from build123d import *

# Parameters (mm, degrees)
SKETCH1_R           = 1
SKETCH1_R_2         = 4.5
BOSS_EXTRUDE1_DEPTH = 2
SKETCH1_4_R         = 4.5
CUT_EXTRUDE1_DEPTH  = 1


with BuildPart() as part:
    # Sketch1 → Boss-Extrude1 (new body)
    with BuildSketch(Plane(origin=(0, 0, 0), x_dir=(1, 0, 0), z_dir=(0, 1, 0))):
        with BuildLine():
            Line((-6, 11), (6, 11))
            ThreePointArc((6, 11), (9.535533906, 9.535533906), (11, 6))
            Line((11, 6), (11, -6))
            ThreePointArc((11, -6), (9.535533906, -9.535533906), (6, -11))
            Line((6, -11), (-6, -11))
            ThreePointArc((-6, -11), (-9.535533906, -9.535533906), (-11, -6))
            Line((-11, -6), (-11, 6))
            ThreePointArc((-11, 6), (-9.535533906, 9.535533906), (-6, 11))
        make_face()
        with Locations((-6.992221877, 6.992221877)):
            Circle(SKETCH1_R, mode=Mode.SUBTRACT)
        with Locations((6.992221877, 6.992221877)):
            Circle(SKETCH1_R, mode=Mode.SUBTRACT)
        with Locations((6.992221877, -6.992221877)):
            Circle(SKETCH1_R, mode=Mode.SUBTRACT)
        with Locations((-6.992221877, -6.992221877)):
            Circle(SKETCH1_R, mode=Mode.SUBTRACT)
        Circle(SKETCH1_R_2, mode=Mode.SUBTRACT)
        with Locations((-6.363961031, 0)):
            Circle(SKETCH1_R, mode=Mode.SUBTRACT)
        with Locations((6.363961031, 0)):
            Circle(SKETCH1_R, mode=Mode.SUBTRACT)
    extrude(amount=BOSS_EXTRUDE1_DEPTH)

    # Sketch1_4 → Cut-Extrude1 (cut)
    with BuildSketch(Plane(origin=(0, 0, 0), x_dir=(1, 0, 0), z_dir=(0, 1, 0))):
        with BuildLine():
            Line((2.121320344, 9.192388155), (9.192388155, 2.121320344))
            ThreePointArc((9.192388155, 2.121320344), (10.071067812, 0), (9.192388155, -2.121320344))
            Line((9.192388155, -2.121320344), (2.121320344, -9.192388155))
            ThreePointArc((2.121320344, -9.192388155), (0, -10.071067812), (-2.121320344, -9.192388155))
            Line((-2.121320344, -9.192388155), (-9.192388155, -2.121320344))
            ThreePointArc((-9.192388155, -2.121320344), (-10.071067812, 0), (-9.192388155, 2.121320344))
            Line((-9.192388155, 2.121320344), (-2.121320344, 9.192388155))
            ThreePointArc((-2.121320344, 9.192388155), (0, 10.071067812), (2.121320344, 9.192388155))
        make_face()
        Circle(SKETCH1_4_R, mode=Mode.SUBTRACT)
    extrude(amount=CUT_EXTRUDE1_DEPTH, mode=Mode.SUBTRACT)


solid = part.part
Can you work these out from the model? Positions are in its coordinate system, mm. A direction names the side the tool comes from. Coordinates: 2 decimals unless noted, no trailing zeros. Order: outer loops, then holes, each group sorted by start corner. A loop starts at its lowest first (then second) coordinate and runs counter-clockwise, first axis right, second up. Notation, with made-up numbers: (-21, -3.75) -> (-2, -3.75) arc R21 ccw to (-2, 35.25) -> close; hole circle Ø3 at (6.25, -4.75). An arc over 180 degrees is marked (long way). Use one line per item in the form item = value.
Q1. Imagine slicing it at B-B, the plane x = 0. List the corners of the cut face in (y, z) for me, then the cut area to 3 significant figures.
From the geometry:
outline = (0, -11) -> (2, -11) -> (2, -4.5) -> (1, -4.5) -> (1, -10.07) -> (0, -10.07) -> close; (0, 10.07) -> (1, 10.07) -> (1, 4.5) -> (2, 4.5) -> (2, 11) -> (0, 11) -> close
area = 14.9 mm²
Q2. I need wall thicknesses on L1, parallel to X at y = 1.7, z = 0; L2, parallel to Z at x = 7.75, y = 1.1; L3, parallel to X at y = 0.8, z = -6.5. Which ranges of each line are inside material? Lowest first, please.
From the geometry:
L1 = -11 to -7.36, -5.36 to -4.5, 4.5 to 5.36, 7.36 to 11
L2 = -10.68 to -7.64, -6.34 to 6.34, 7.64 to 10.68
L3 = -10.97 to -7.86, -6.12 to -4.81, 4.81 to 6.12, 7.86 to 10.97
Q3. Will these pins go through, and if not, where does the flat tip stop? P1, Ø10.5, axis at x = 0, z = 0, coming from the -Y side; P2, Ø1.2, axis at x = 6.99, z = 6.99, coming from the +Y side.
From the geometry:
P1 = 1
P2 = through
Q4. Imagine slicing it at C-C, the plane z = 3. List the corners of the cut face in (x, y) for me, then the cut area to 3 significant figures.
From the geometry:
outline = (-11, 0) -> (-8.31, 0) -> (-8.31, 1) -> (-3.35, 1) -> (-3.35, 2) -> (-11, 2) -> close; (3.35, 1) -> (8.31, 1) -> (8.31, 0) -> (11, 0) -> (11, 2) -> (3.35, 2) -> close
area = 20.7 mm²
Q5. Imagine slicing it at A-A, the plane z = 0. List the corners of the cut face in (x, y) for me, then the cut area to 3 significant figures.
From the geometry:
outline = (-11, 0) -> (-10.07, 0) -> (-10.07, 1) -> (-7.36, 1) -> (-7.36, 2) -> (-11, 2) -> close; (-5.36, 1) -> (-4.5, 1) -> (-4.5, 2) -> (-5.36, 2) -> close; (4.5, 1) -> (5.36, 1) -> (5.36, 2) -> (4.5, 2) -> close; (7.36, 1) -> (10.07, 1) -> (10.07, 0) -> (11, 0) -> (11, 2) -> (7.36, 2) -> close
area = 10.9 mm²
Q6. Imagine slicing it at D-D, the plane x = -7. List the corners of the cut face in (y, z) for me, then the cut area to 3 significant figures.
From the geometry:
outline = (0, -10.9) -> (2, -10.9) -> (2, -7.99) -> (0, -7.99) -> close; (0, -5.99) -> (2, -5.99) -> (2, -0.77) -> (1, -0.77) -> (1, -4.31) -> (0, -4.31) -> close; (0, 4.31) -> (1, 4.31) -> (1, 0.77) -> (2, 0.77) -> (2, 5.99) -> (0, 5.99) -> close; (0, 7.99) -> (2, 7.99) -> (2, 10.9) -> (0, 10.9) -> close
area = 25.4 mm²
Q7. Which directions (+Z, -Z, +X, -X, +Y, -Y) give clear straight access to the entire face, cutting with the end or side of a thin tool? Please do faces 4 (the face through (6.2, 0.99, -6.38)), 5 (the face through (-5.706, 0.493, -5.607)).
From the geometry:
face_4 = +Y, -Y
face_5 = -Y
Q8. We'd pull the mould along Z, two halves only. Please class faces 1 (the face through (10.07, 0.49, -0.03)), 2 (the face through (7, 0, 5)), 3 (the face through (9, 1, -10)): released by +Z, released by -Z, zero draft, split by the parting line, or undercut.
From the geometry:
face_1 = undercut
face_2 = zero draft
face_3 = released by -Z
